Read the model definition and answer for the solid it produces. Units are mm, in the model's axes. Give positions to 0.01 mm unless a question says otherwise; leave off trailing zeros. Write each loop counter-clockwise with the first axis right and the second up, starting at its lowest first coordinate (ties: lowest second). Pieces come first, ordered by that corner, then holes. Notation, with made-up numbers: (68, 15.5) -> (98, 15.5) arc R24 ccw to (98, 33.5) -> close; hole circle Ø9 at (72.5, -10.5). An arc over 180 degrees is marked (long way). Write item = value, one per line.
from build123d import *

# Parameters (mm, degrees)
SKETCH1_W           = 15
SKETCH1_H           = 15
SKETCH1_R           = 4.05
BOSS_EXTRUDE1_DEPTH = 30
SKETCH2_R           = 1.75
CUT_EXTRUDE1_DEPTH  = 35.369317712


with BuildPart() as part:
    # Sketch1 → Boss-Extrude1 (new body)
    with BuildSketch(Plane.XY):
        Rectangle(SKETCH1_W, SKETCH1_H)
        Circle(SKETCH1_R, mode=Mode.SUBTRACT)
    extrude(amount=BOSS_EXTRUDE1_DEPTH)

    # Sketch2 → Cut-Extrude1 (cut, through all)
    with BuildSketch(Plane(origin=(0, 7.5, 0), x_dir=(1, 0, 0), z_dir=(0, 1, 0))):
        with Locations((7.5, -30)):
            Circle(SKETCH2_R)
        with Locations((7.5, 0)):
            Circle(SKETCH2_R)
        with Locations((-7.5, 0)):
            Circle(SKETCH2_R)
        with Locations((-7.5, -30)):
            Circle(SKETCH2_R)
    extrude(amount=-CUT_EXTRUDE1_DEPTH, mode=Mode.SUBTRACT)


solid = part.part
(1) The part is cut by section A-A on x = 0. Determine the outline of the cut face in (y, z), plus the area to 3 significant figures.
Checks:
outline = (-7.5, 0) -> (-4.05, 0) -> (-4.05, 30) -> (-7.5, 30) -> close; (4.05, 0) -> (7.5, 0) -> (7.5, 30) -> (4.05, 30) -> close
area = 207 mm²
(2) The part is cut by section D-D on z = 8.75. Determine the outline of the cut face in (x, y).
Checks:
outline = (-7.5, -7.5) -> (7.5, -7.5) -> (7.5, 7.5) -> (-7.5, 7.5) -> close; hole circle Ø8.1 at (0, 0)
(3) For a pull along Y with two mould halves and no side action, classify faces 1 (the cylindrical face through (-0.878, -3.954, 14.79)), 2 (the flat face through (0, -7.5, 15)), 3 (the cylindrical face through (6.276, 0.105, 28.749)) as released by +Y, released by -Y, zero draft, split by the parting line, or undercut.
Checks:
face_1 = undercut
face_2 = released by -Y
face_3 = zero draft
(4) Consider L1, parallel to Y at x = 0, z = 14.5; L2, parallel to X at y = -1, z = 14; L3, parallel to X at y = 3.5, z = 7.5. Determine where each line is inside the solid, lowest interval first.
Checks:
L1 = -7.5 to -4.05, 4.05 to 7.5
L2 = -7.5 to -3.92, 3.92 to 7.5
L3 = -7.5 to -2.04, 2.04 to 7.5
(5) The part is cut by section B-B on y = 0. Determine the outline of the cut face in (x, z), plus the area to 3 significant figures.
Checks:
outline = (-7.5, 1.75) arc R1.75 cw to (-5.75, 0) -> (-4.05, 0) -> (-4.05, 30) -> (-5.75, 30) arc R1.75 cw to (-7.5, 28.25) -> close; (4.05, 0) -> (5.75, 0) arc R1.75 cw to (7.5, 1.75) -> (7.5, 28.25) arc R1.75 cw to (5.75, 30) -> (4.05, 30) -> close
area = 197 mm²
(6) Given P1, Ø2, axis at x = -2, y = -2.5, coming from the +Z side, flat-ended and moving along its own axis, determine where the tip first touches the part or whether it passes through.
Checks:
P1 = 30
(7) The part is cut by section C-C on y = 4.75. Determine the outline of the cut face in (x, z), plus the area to 3 significant figures.
Checks:
outline = (-7.5, 1.75) arc R1.75 cw to (-5.75, 0) -> (5.75, 0) arc R1.75 cw to (7.5, 1.75) -> (7.5, 28.25) arc R1.75 cw to (5.75, 30) -> (-5.75, 30) arc R1.75 cw to (-7.5, 28.25) -> close
area = 440 mm²
